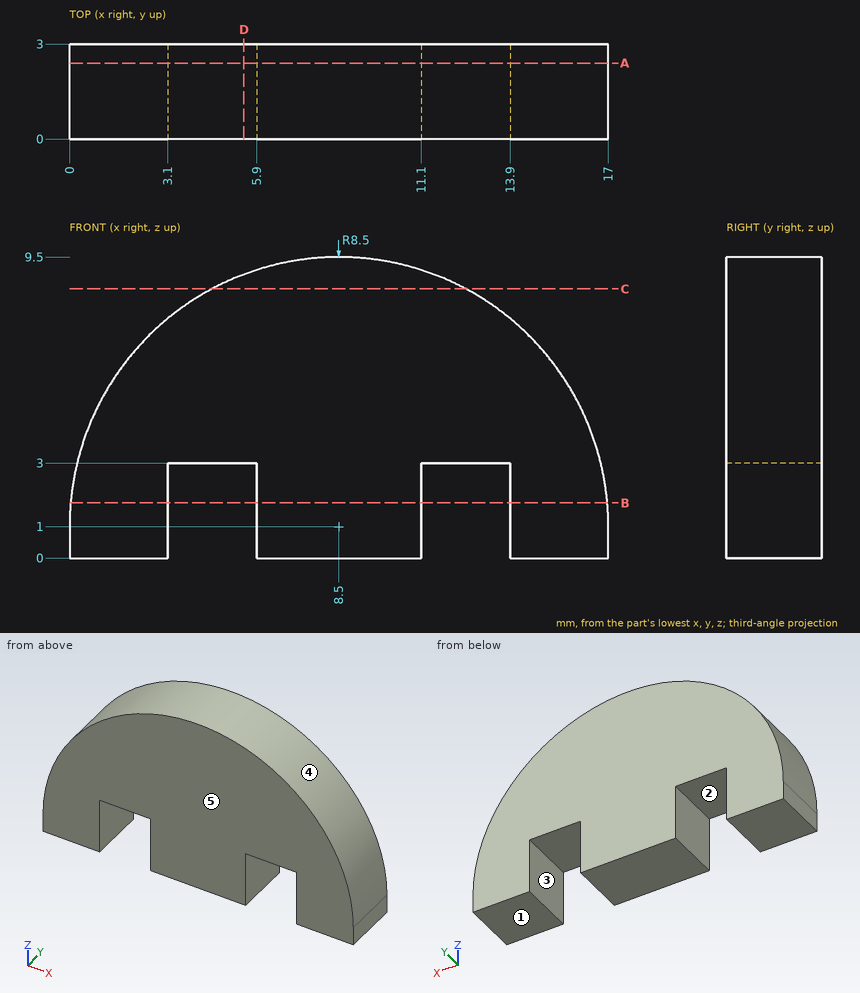
The drawing under review shows one solid part. Ordinate dimensions are in mm from its lowest x, y, z. A direction names the side the tool comes from. Coordinates: 2 decimals unless noted, no trailing zeros. Write each loop counter-clockwise with the first axis right and the second up, starting at its lowest first coordinate (ties: lowest second). Pieces come first, ordered by that corner, then holes. Notation, with made-up numbers: (46.25, 67) - (76.25, 67) arc R25 cw to (76.25, 102) - close; hole circle Ø11 at (39, 71.5). An arc over 180 degrees is marked (long way). Put each result on its own line as item: value.
1. Mouldability with a two-part tool opening along X and no side actions: class the marked faces 3, 4 and 5 as released by +X, released by -X, zero draft, split by the parting line, or undercut.
Values found:
face 3: undercut
face 4: split by the parting line
face 5: zero draft
2. Add section D-D, the plane x = 5.5. Give the boundary of the cut face in (y, z).
Values found:
outline: (0, 3) - (3, 3) - (3, 8.95) - (0, 8.95) - close
3. Add section C-C, the plane z = 8.5. Give the boundary of the cut face in (x, y), then the cut area to 3 significant figures.
Values found:
outline: (4.5, 0) - (12.5, 0) - (12.5, 3) - (4.5, 3) - close
area: 24.0 mm²
4. For pin 1 (0.9 mm diameter, centred on y = 1.5, z = 2, fed in from -X); pin 2 (0.8 mm diameter, centred on x = 12.5, y = 2, fed in from -Z), all flat-tipped, find the tip position at first contact; note any pin that passes through.
Values found:
pin 1: x = 0.02
pin 2: z = 3
5. Wall thickness on probe 1 along X at (y, z) = (2.15, 1.25); probe 2 along X at (y, z) = (0.9, 2); probe 3 along Z at (x, y) = (8.25, 0.85): over which ranges is each line inside the solid? List them lowest first.
Values found:
probe 1: 0 to 3.1, 5.9 to 11.1, 13.9 to 17
probe 2: 0.06 to 3.1, 5.9 to 11.1, 13.9 to 16.94
probe 3: 0 to 9.5
6. Add section B-B, the plane z = 1.75. Give the boundary of the cut face in (x, y).
Values found:
outline: (0.03, 0) - (3.1, 0) - (3.1, 3) - (0.03, 3) - close; (5.9, 0) - (11.1, 0) - (11.1, 3) - (5.9, 3) - close; (13.9, 0) - (16.97, 0) - (16.97, 3) - (13.9, 3) - close
7. Add section A-A, the plane y = 2.4. Give the boundary of the cut face in (x, z).
Values found:
outline: (0, 0) - (3.1, 0) - (3.1, 3) - (5.9, 3) - (5.9, 0) - (11.1, 0) - (11.1, 3) - (13.9, 3) - (13.9, 0) - (17, 0) - (17, 1) arc R8.5 ccw to (0, 1) - close
8. Machinability: for the marked faces 1 and 2, which of the approach directions +Z, -Z, +X, -X, +Y, -Y give a long, thin tool a straight path to every point of the face, cutting with its end or side? Answer none if there is none.
Values found:
face 1: -Z, +X, -X, +Y, -Y
face 2: -Z, +Y, -Y
